Design review of the part built by this model. Coordinates are the model's own, in mm. A direction names the side the tool comes from. Coordinates: 2 decimals unless noted, no trailing zeros. Order: outer loops, then holes, each group sorted by start corner. A loop starts at its lowest first (then second) coordinate and runs counter-clockwise, first axis right, second up. Notation, with made-up numbers: (22.25, -6.5) -> (75.25, -6.5) arc R16 ccw to (75.25, 1.5) -> close; hole circle Ø11 at (36.25, -36.75). An arc over 180 degrees is marked (long way). Write item = value, one per line.
```python
from build123d import *

# Parameters (mm, degrees)
SKETCH1_W           = 120
SKETCH1_H           = 120
BOSS_EXTRUDE1_DEPTH = 50
SKETCH2_R           = 35
BOSS_EXTRUDE2_DEPTH = 25
SKETCH3_R           = 25
CUT_EXTRUDE1_DEPTH  = 186.539753153
FILLET1_R           = 10
FILLET2_R           = 1.5
SHELL1_T            = -2


with BuildPart() as part:
    # Sketch1 → Boss-Extrude1 (new body)
    with BuildSketch(Plane.XY):
        with Locations((60, 60)):
            Rectangle(SKETCH1_W, SKETCH1_H)
    extrude(amount=BOSS_EXTRUDE1_DEPTH)

    # Sketch2 → Boss-Extrude2 (add)
    with BuildSketch(Plane.XY.offset(50)):
        with Locations(Location((60, 60, 0), (0, 0, 180))):
            Circle(SKETCH2_R)
    extrude(amount=BOSS_EXTRUDE2_DEPTH)

    # Sketch3 → Cut-Extrude1 (cut, through all)
    with BuildSketch(Plane.XY.offset(75)):
        with Locations((60, 60)):
            Circle(SKETCH3_R)
    extrude(amount=-CUT_EXTRUDE1_DEPTH, mode=Mode.SUBTRACT)

    # Fillet1
    fillet1_edges = [part.edges().sort_by_distance(p)[0] for p in [
        (0, 120, 25),
        (120, 120, 25),
        (120, 0, 25),
        (0, 0, 25),
    ]]
    fillet(fillet1_edges, radius=FILLET1_R)

    # Fillet2
    fillet2_edges = [part.edges().sort_by_distance(p)[0] for p in [
        (95, 60, 75),
        (35, 60, 75),
    ]]
    fillet(fillet2_edges, radius=FILLET2_R)

    # Shell1
    shell1_openings = [part.faces().sort_by_distance(p)[0] for p in [
        (60, 1.697056275, 0),
    ]]
    offset(amount=SHELL1_T, openings=shell1_openings, kind=Kind.INTERSECTION)


solid = part.part
```
(1) For L1, parallel to Y at x = 60, z = 41.5; L2, parallel to X at y = 59.5, z = 38 (3 decimals); L3, parallel to Y at x = 67.5, z = 65.5, list the stretches that pass through material, from the lowest coordinate up.
Report:
L1 = 0 to 2, 33 to 35, 85 to 87, 118 to 120
L2 = 0 to 2, 33.005 to 35.005, 84.995 to 86.995, 118 to 120
L3 = 25.81 to 27.86, 34.06 to 36.15, 83.85 to 85.94, 92.14 to 94.19
(2) Insertion check: pin 1 (5 mm diameter, centred on x = 35.5, y = 100, fed in from +Z); pin 2 (1 mm diameter, centred on x = 75.5, y = 91.5, fed in from +Z); pin 3 (8 mm diameter, centred on x = 88, y = 21.5, fed in from -Z). Each pin has a flat end and moves straight along its axis. Give the tip position at first contact, or say it passes through.
Report:
pin_1 = 50
pin_2 = 74.51
pin_3 = 48
(3) The part is to be moulded in two halves that separate along Y. For faces 3 (the cylindrical face through (115.594, 115.719, 24.336)), 4 (the cylindrical face through (41.18, 30.49, 61.59)), 5 (the flat face through (84, 52, 0)), 6 (the cylindrical face through (84.94, 49.66, 37.01)), say which applies: released by +Y, released by -Y, zero draft, split by the parting line, or undercut.
Report:
face_3 = undercut
face_4 = split by the parting line
face_5 = zero draft
face_6 = undercut
(4) We need section D-D (y = 12). Write out the cut boundary in (x, z), and give its area (3 significant figures).
Report:
outline = (0, 0) -> (2, 0) -> (2, 48) -> (118, 48) -> (118, 0) -> (120, 0) -> (120, 50) -> (0, 50) -> close
area = 432 mm²
(5) We need section B-B (x = 60). Write out the cut boundary in (y, z), and give its area (3 significant figures).
Report:
outline = (0, 0) -> (2, 0) -> (2, 48) -> (27, 48) -> (27, 73) -> (33, 73) -> (33, 0) -> (35, 0) -> (35, 73.5) arc R1.5 ccw to (33.5, 75) -> (26.5, 75) arc R1.5 ccw to (25, 73.5) -> (25, 50) -> (0, 50) -> close; (85, 0) -> (87, 0) -> (87, 73) -> (93, 73) -> (93, 48) -> (118, 48) -> (118, 0) -> (120, 0) -> (120, 50) -> (95, 50) -> (95, 73.5) arc R1.5 ccw to (93.5, 75) -> (86.5, 75) arc R1.5 ccw to (85, 73.5) -> close
area = 722 mm²
(6) We need section A-A (z = 37.5). Write out the cut boundary in (x, y).
Report:
outline = (0, 10) arc R10 ccw to (10, 0) -> (110, 0) arc R10 ccw to (120, 10) -> (120, 110) arc R10 ccw to (110, 120) -> (10, 120) arc R10 ccw to (0, 110) -> close; circle Ø54 at (60, 60); hole (2, 10) arc R8 ccw to (10, 2) -> (110, 2) arc R8 ccw to (118, 10) -> (118, 110) arc R8 ccw to (110, 118) -> (10, 118) arc R8 ccw to (2, 110) -> close; hole circle Ø50 at (60, 60)
(7) For faces 1 (the flat face through (59, 118, 24)), 2 (the flat face through (59, 0, 25)), list the 3-axis set-ups (+Z, -Z, +X, -X, +Y, -Y) from which the entire face can be reached by the end or side of a thin tool; tool diameter is ignored.
Report:
face_1 = -Z
face_2 = +Z, -Z, +X, -X, -Y
